Build history of the part. All positions in model axes, mm. Face numbers are marked on the shaded views. A direction names the side the tool comes from. Round coordinates to 2 decimals unless told otherwise and drop trailing zeros. Write each loop counter-clockwise with the first axis right and the second up, starting at its lowest first coordinate (ties: lowest second). Pieces come first, ordered by that corner, then holes. Notation, with made-up numbers: M 68,-22 L 106,-22 A18 cw 106,-1 Z; hole C 18,63 d5. An arc over 180 degrees is marked long. Write item = value, one per line.
from build123d import *

# Parameters (mm, degrees)
EXTRUDE_1_DEPTH     = 22
SKETCH_2_R          = 1.1
CUT_EXTRUDE_1_DEPTH = 22
CUT_EXTRUDE_2_DEPTH = 4
FILLET_2_R          = 1
EXTRUDE_2_DEPTH     = 6
EXTRUDE_3_DEPTH     = 6


with BuildPart() as part:
    # 草图1 → 凸台-拉伸1 (new body)
    with BuildSketch(Plane.XY):
        with BuildLine():
            Line((0, 0), (28, 0))
            ThreePointArc((28, 0), (19.798989873, -19.798989873), (0, -28))
            Line((0, -28), (0, 0))
        make_face()
    extrude(amount=EXTRUDE_1_DEPTH)

    # 草图2 → 切除-拉伸1 (cut)
    with BuildSketch(Plane.XY.offset(22)):
        with Locations((2, -2)):
            Circle(SKETCH_2_R)
        with Locations((26, -2)):
            Circle(SKETCH_2_R)
        with Locations(Location((2, -26, 0), (0, 0, 180))):
            Circle(SKETCH_2_R)
    extrude(amount=-CUT_EXTRUDE_1_DEPTH, mode=Mode.SUBTRACT)

    # 草图4 → 切除-拉伸2 (cut)
    with BuildSketch(Plane.XY.offset(22)):
        with BuildLine():
            Line((4.5, -2), (4.5, 0.5))
            Line((4.5, 0.5), (-2.867094288, 0.5))
            Line((-2.867094288, 0.5), (-2.867094288, -4.5))
            Line((-2.867094288, -4.5), (2, -4.5))
            ThreePointArc((2, -4.5), (3.767766953, -3.767766953), (4.5, -2))
        make_face()
    extrude(amount=-CUT_EXTRUDE_2_DEPTH, mode=Mode.SUBTRACT)

    # 圆角2
    fillet_2_edges = [part.edges().sort_by_distance(p)[0] for p in [
        (0, 0, 9),
        (28, 0, 11),
        (0, -28, 11),
    ]]
    fillet(fillet_2_edges, radius=FILLET_2_R)

    # 草图5 → 凸台-拉伸2 (add)
    with BuildSketch(Plane.ZY):
        with BuildLine():
            Line((0, -9.19490604), (0, -18.786569087))
            ThreePointArc((0, -18.786569087), (11, -25.990737563), (22, -18.786569087))
            Line((22, -18.786569087), (22, -9.19490604))
            ThreePointArc((22, -9.19490604), (11, -1.990737563), (0, -9.19490604))
        make_face()
    extrude(amount=EXTRUDE_2_DEPTH)

    # 草图6 → 凸台-拉伸3 (add)
    with BuildSketch(Plane(origin=(0, 0, 0), x_dir=(1, 0, 0), z_dir=(0, 1, 0))):
        with BuildLine():
            Line((9.19490604, 0), (18.786569087, 0))
            ThreePointArc((18.786569087, 0), (25.990737563, -11), (18.786569087, -22))
            Line((18.786569087, -22), (9.19490604, -22))
            ThreePointArc((9.19490604, -22), (1.990737563, -11), (9.19490604, 0))
        make_face()
    extrude(amount=EXTRUDE_3_DEPTH)


solid = part.part
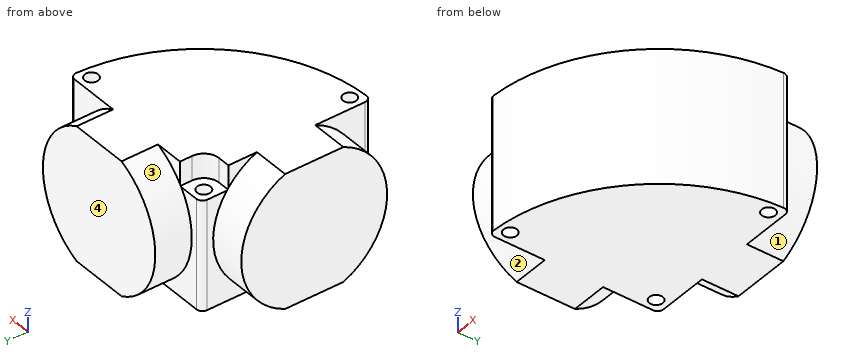
1. Tool access for the marked faces 1, 2, 3 and 4: list every direction of +Z, -Z, +X, -X, +Y, -Y with a clear straight run to the whole face (end or side of a thin tool).
Responses:
face_1 = +X, +Y
face_2 = -X, -Y
face_3 = -X, +Y
face_4 = +Z, -Z, +X, -X, +Y
2. Band-saw the part on B-B (x = 7.5). List the corners of the cut face in (y, z).
Responses:
outline = M -26.98,0 L 0,0 L 0,0.91 L 6,0.91 L 6,21.09 L 0,21.09 L 0,22 L -26.98,22 Z
3. Flat gauge pins, fed straight in: pin 1 (3.5 mm diameter, centred on x = 26, y = -2, fed in from -Z); pin 2 (2 mm diameter, centred on y = -11.5, z = 4, fed in from +X); pin 3 (1.3 mm diameter, centred on x = 1.5, y = -1, fed in from +Z); pin 4 (1.5 mm diameter, centred on y = 0, z = 9, fed in from -X). Where does each tip first touch, or does it go through?
Responses:
pin_1 = 0
pin_2 = 25.96
pin_3 = 18
pin_4 = 0.03
4. Band-saw the part on C-C (y = 1). List the corners of the cut face in (x, z).
Responses:
outline = M 9.19,0 L 18.79,0 A12 ccw 18.79,22 L 9.19,22 A12 ccw Z
5. Band-saw the part on D-D (z = 16). List the corners of the cut face in (x, y), plus the area to 3 significant figures.
Responses:
outline = M -6,-24.9 L 0,-24.9 L 0,-26.98 A1 ccw 1.04,-27.98 A28 ccw 27.98,-1.04 A1 ccw 26.98,0 L 24.9,0 L 24.9,6 L 3.08,6 L 3.08,0 L 1,0 A1 ccw 0,-1 L 0,-3.08 L -6,-3.08 Z; hole C 2,-26 d2.2; hole C 2,-2 d2.2; hole C 26,-2 d2.2
area = 865 mm²
6. Band-saw the part on A-A (z = 9). List the corners of the cut face in (x, y).
Responses:
outline = M -6,-25.82 L 0,-25.82 L 0,-26.98 A1 ccw 1.04,-27.98 A28 ccw 27.98,-1.04 A1 ccw 26.98,0 L 25.82,0 L 25.82,6 L 2.16,6 L 2.16,0 L 1,0 A1 ccw 0,-1 L 0,-2.16 L -6,-2.16 Z; hole C 2,-26 d2.2; hole C 2,-2 d2.2; hole C 26,-2 d2.2
7. Probe probe 1 along Z at (x, y) = (4, -3); probe 2 along Y at (x, z) = (2, 5); probe 3 along X at (y, z) = (-26, 12.5). List the from-to ranges inside material, lowest first.
Responses:
probe_1 = 0 to 18
probe_2 = -27.93 to -27.1, -24.9 to -3.1, -0.9 to 0
probe_3 = 0 to 0.9, 3.1 to 10.39
